```python
from build123d import *

# Parameters (mm, degrees)
F1_DEPTH = 76.2
F2_SIZE  = 12.7
F3_SIZE  = 45.72


with BuildPart() as f1:
    # F0 (on Top) → F1 (new body)
    with BuildSketch(Plane.XY):
        Polygon((-22.704043, 43.176515), (-43.746475, 21.585433), (-48.079241, -8.250551), (-34.047371, -34.935105), (-7.010562, -48.275636), (22.704043, -43.176515), (43.746475, -21.585433), (48.079241, 8.250551), (34.047371, 34.935105), (7.010562, 48.275636), align=None)
    extrude(amount=F1_DEPTH)

    # F2
    f2_edges = [f1.edges().sort_by_distance(p)[0] for p in [
        (7.84674, -45.726075, 76.2),
        (33.225259, -32.380974, 76.2),
        (45.912858, -6.667441, 76.2),
        (41.063306, 21.592828, 76.2),
        (20.528967, 41.60537, 76.2),
        (-7.84674, 45.726075, 76.2),
        (-20.528967, -41.60537, 76.2),
        (-41.063306, -21.592828, 76.2),
        (-45.912858, 6.667441, 76.2),
        (-33.225259, 32.380974, 76.2),
    ]]
    chamfer(f2_edges, length=F2_SIZE)

    # F3
    f3_edges = [f1.edges().sort_by_distance(p)[0] for p in [
        (-20.528967, -41.60537, 0),
        (7.84674, -45.726075, 0),
        (33.225259, -32.380974, 0),
        (45.912858, -6.667441, 0),
        (41.063306, 21.592828, 0),
        (20.528967, 41.60537, 0),
        (-7.84674, 45.726075, 0),
        (-33.225259, 32.380974, 0),
        (-45.912858, 6.667441, 0),
        (-41.063306, -21.592828, 0),
    ]]
    chamfer(f3_edges, length=F3_SIZE)


solid = f1.part
```
Input: part model. Units: mm. Frame: model coordinates. Round coordinates to 2 decimals unless told otherwise and drop trailing zeros. Loops run counter-clockwise (first coordinate to the right, second up) from the corner with the lowest first, then second, coordinate; pieces in that order, holes last. Notation, with made-up numbers: (15, 47.5) -> (72, 47.5) arc R13 ccw to (72, 66.5) -> close; hole circle Ø1 at (33, -1.75). An arc over 180 degrees is marked (long way). Use one line per item in the form item = value. Start each with the question number.
Item 1: Contact query for flat-ended pins moving along their axis: pin 1 Ø6 at (x, y) = (7, 4) entering from -Z; pin 2 Ø6 at (x, y) = (-31, 23) entering from -Z; pin 3 Ø3 at (y, z) = (11.5, 60.5) entering from -X. Output: stop coordinate, or through.
Item 2: Section query D-D on z = 39. Return the cut outline in (x, y), then the cut area to 3 significant figures.
Item 3: Section query A-A on z = 52. Return the cut outline in (x, y), then the cut area to 3 significant figures.
Item 4: Section query B-B on x = 41.5. Return the cut outline in (y, z).
Item 5: Section query C-C on y = -2.5. Return the cut outline in (x, z).
Item 6: Material intervals for L1, parallel to Y at x = 27.5, z = 37; L2, parallel to X at y = 0, z = 9; L3, parallel to Z at x = 19.5, y = -10, sorted ascending. Write a range as from..to.
Ans:
q1.pin_1 = 4.38
q1.pin_2 = 34.58
q1.pin_3 = -45.43
q2.outline = (-41.12, -7.06) -> (-29.12, -29.87) -> (-6, -41.28) -> (19.42, -36.92) -> (37.41, -18.46) -> (41.12, 7.06) -> (29.12, 29.87) -> (6, 41.28) -> (-19.42, 36.92) -> (-37.41, 18.46) -> close
q2.area = 5,110 mm^2
q3.outline = (-48.08, -8.25) -> (-34.05, -34.94) -> (-7.01, -48.28) -> (22.7, -43.18) -> (43.75, -21.59) -> (48.08, 8.25) -> (34.05, 34.94) -> (7.01, 48.28) -> (-22.7, 43.18) -> (-43.75, 21.59) -> close
q3.area = 6,990 mm^2
q4.outline = (-23.89, 45.72) -> (-20.48, 43.34) -> (7.12, 39.37) -> (20.76, 45.72) -> (20.76, 63.5) -> (7.12, 69.85) -> (-20.48, 65.88) -> (-23.89, 63.5) -> close
q5.outline = (-47.24, 45.72) -> (-14.57, 13.38) -> (-2.44, 2.65) -> (-0.36, 1.73) -> (1.31, 2.01) -> (5.07, 4.7) -> (46.52, 45.72) -> (46.52, 63.5) -> (33.68, 76.2) -> (-34.41, 76.2) -> (-47.24, 63.5) -> close
q6.L1 = -25.76..28.44
q6.L2 = -9.78..9.78
q6.L3 = 20.27..76.2
